Geometry check sheet. Reference: the model listing, model coordinates, mm. A direction names the side the tool comes from. Round coordinates to 2 decimals unless told otherwise and drop trailing zeros. Loops run counter-clockwise (first coordinate to the right, second up) from the corner with the lowest first, then second, coordinate; pieces in that order, holes last. Notation, with made-up numbers: (10.25, -29.5) -> (35.25, -29.5) arc R13 cw to (35.25, -15.5) -> close; hole circle Ø7 at (67, 18). An arc over 180 degrees is marked (long way). Use a Markdown table: item, result. Add a question column.
Q1. Sectioned sample at B-B, the plane y = -15. Give the number of separate pieces and of enclosed holes in the cut face, then the cut area to 3 significant figures.
Q2. Gauge pin test, flat ends, axial feed: P1, Ø2, axis at y = -10.5, z = 1, coming from the +X side; P2, Ø0.8, axis at y = -20.5, z = 0, coming from the -X side; P3, Ø2, axis at y = -21, z = 0, coming from the +X side. Record the tip position at first contact, or that the pin passes through.
Q3. Release check for a two-part mould opening along Y. For faces 1 (the face through (0, -22.434, 0)), 2 (the face through (4, -22, 0)), 3 (the face through (0, -8.03, 0)) record: released by +Y, released by -Y, zero draft, split by the parting line, or undercut.
Q4. Material ranges on L1, parallel to X at y = -11.5, z = -1.05; L2, parallel to X at y = -2, z = -1; L3, parallel to Y at x = 4.5, z = 1.4, recorded low to high.
Q5. Sectioned sample at A-A, the plane z = -0.55. Enter the section's corners in (x, y).
Q6. Set-up check for faces 4 (the face through (-4, -22, 0)), 5 (the face through (0, -14, 2)): record each of +Z, -Z, +X, -X, +Y, -Y from which the full face is reachable in a straight line by a thin tool's end or side.
```python
from build123d import *

# Parameters (mm, degrees)
F1_R          = 2.00017
F4_DEPTH      = 2
F4_DEPTH_BACK = 2


with BuildPart() as f2:
    # F2: sweep along a path in F0
    with BuildLine(Plane.XY) as f2_path:
        CenterArc((0, 0), 18, 0, 360)
    # F1 (on Front) → F2 (sweep)
    with BuildSketch(Plane.XZ):
        with Locations((-20.043772, 0)):
            Circle(F1_R)
    sweep(path=f2_path.line)

    # F3 (on Top) → F4 (join, two sides)
    with BuildSketch(Plane.XY) as f4_sk:
        Polygon((4, -8.030277), (0, -8.030277), (-4, -8.030277), (-4, -19.934135), (-4, -22.434135), (4, -22.434135), (4, -19.934135), align=None)
    extrude(amount=F4_DEPTH)
    extrude(f4_sk.sketch, amount=-F4_DEPTH_BACK)


solid = f2.part
```
Values:
| question | item | result |
|---|---|---|
| 1 | separate pieces | 3 |
| 1 | enclosed holes | 0 |
| 1 | area | 70.3 mm^2 |
| 2 | P1 | x = 19.76 |
| 2 | P2 | x = -9.05 |
| 2 | P3 | x = 9.27 |
| 3 | face 1 | released by -Y |
| 3 | face 2 | zero draft |
| 3 | face 3 | undercut |
| 4 | L1 | -18.46 to -14.29, -4 to 4, 14.29 to 18.46 |
| 4 | L2 | -21.68 to -18.2, 18.2 to 21.68 |
| 4 | L3 | -21 to -18.06, 18.06 to 21 |
| 5 | outline | (-4, -22.43) -> (4, -22.43) -> (4, -21.6) arc R21.97 ccw (long way) to (-4, -21.6) -> close; hole (-4, -17.67) -> (-4, -8.03) -> (4, -8.03) -> (4, -17.67) arc R18.12 ccw (long way) to start |
| 6 | face 4 | -X, -Y |
| 6 | face 5 | +Z, +X, -X, +Y, -Y |
